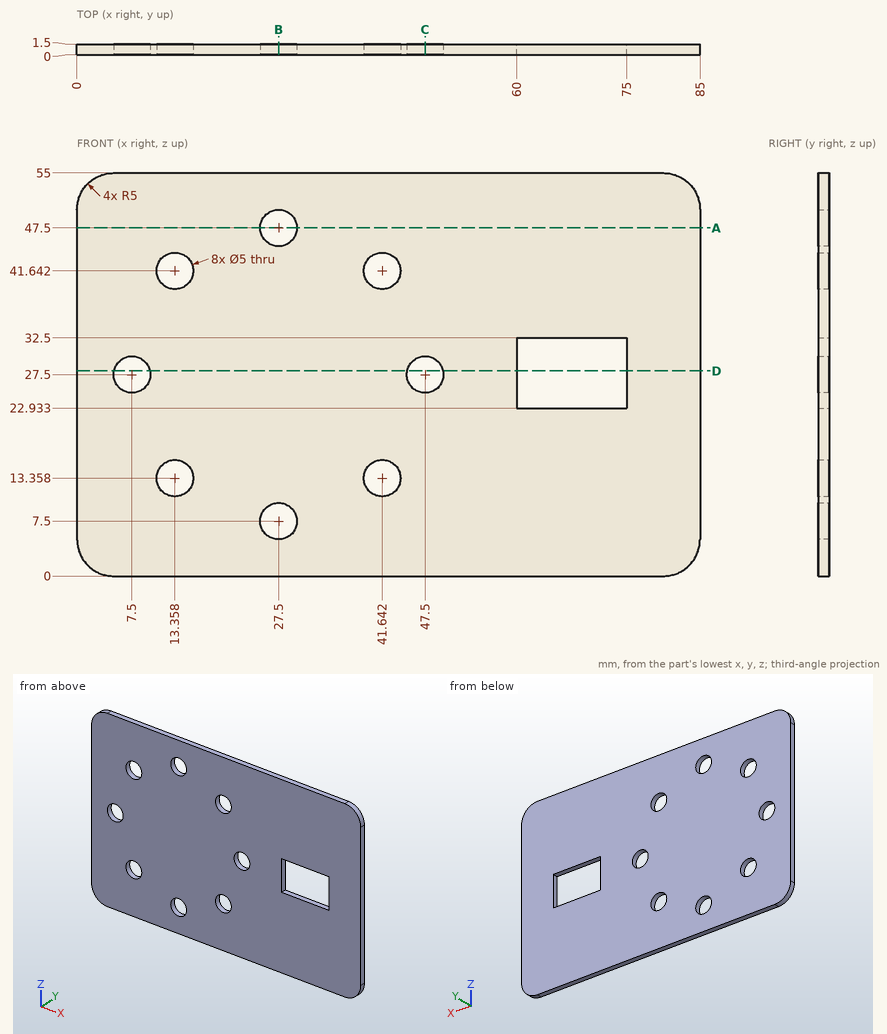
Check sheet for the drawn part. Datum: minimum x, y, z corner. Units: mm. Give positions to 0.01 mm unless a question says otherwise; leave off trailing zeros. Loops run counter-clockwise (first coordinate to the right, second up) from the corner with the lowest first, then second, coordinate; pieces in that order, holes last. Notation, with made-up numbers: M 52,-13 L 62,-13 A24 cw 62,9 Z; hole C 29,67.25 d3. An arc over 180 degrees is marked long. Answer as CSV lines item,"result".
Item 1: Sectioned sample at A-A, the plane z = 47.5. Enter the section's corners in (x, y), then the cut area to 3 significant figures.
Reply:
outline,"M 0,0 L 25,0 L 25,1.5 L 0,1.5 Z; M 30,0 L 85,0 L 85,1.5 L 30,1.5 Z"
area,"120 mm^2"
Item 2: Sectioned sample at D-D, the plane z = 28. Enter the section's corners in (x, y).
Reply:
outline,"M 0,0 L 5.05,0 L 5.05,1.5 L 0,1.5 Z; M 9.95,0 L 45.05,0 L 45.05,1.5 L 9.95,1.5 Z; M 49.95,0 L 60,0 L 60,1.5 L 49.95,1.5 Z; M 75,0 L 85,0 L 85,1.5 L 75,1.5 Z"
Item 3: Depth check by flat-ended pin: pin 1 Ø3 at (x, z) = (47.5, 27.5) entering from -Y; pin 2 Ø6.5 at (x, z) = (13.36, 13.36) entering from -Y. Enter the tip coordinate at first touch or a pass-through.
Reply:
pin 1,"through"
pin 2,"y = 0"
Item 4: Sectioned sample at C-C, the plane x = 47.5. Enter the section's corners in (y, z).
Reply:
outline,"M 0,0 L 1.5,0 L 1.5,25 L 0,25 Z; M 0,30 L 1.5,30 L 1.5,55 L 0,55 Z"
Item 5: Sectioned sample at B-B, the plane x = 27.5. Enter the section's corners in (y, z).
Reply:
outline,"M 0,0 L 1.5,0 L 1.5,5 L 0,5 Z; M 0,10 L 1.5,10 L 1.5,45 L 0,45 Z; M 0,50 L 1.5,50 L 1.5,55 L 0,55 Z"
Item 6: Scan lines: L1, parallel to Z at x = 7.5, y = 0.8; L2, parallel to X at y = 1.15, z = 7.5; L3, parallel to X at y = 1, z = 28.5. Record each from-to range of solid material in increasing order.
Reply:
L1,"0 to 25, 30 to 55"
L2,"0 to 25, 30 to 85"
L3,"0 to 5.21, 9.79 to 45.21, 49.79 to 60, 75 to 85"
